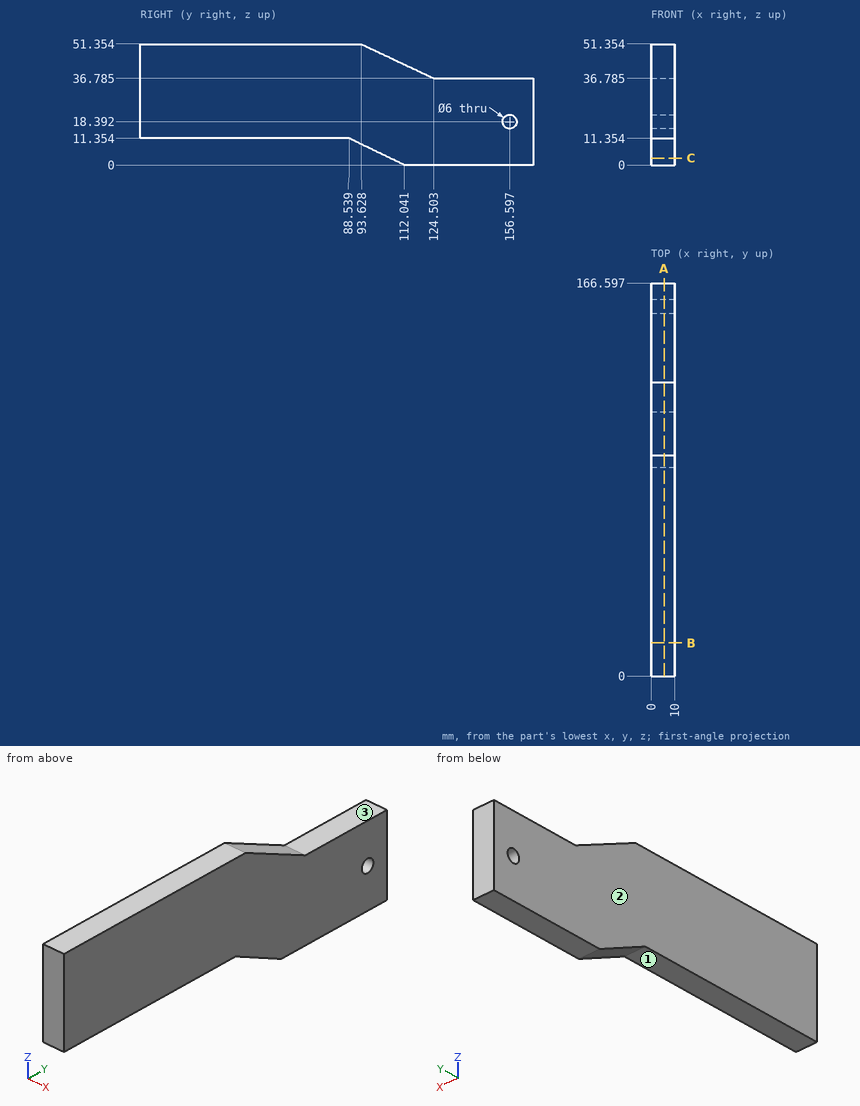
Geometry check sheet. Reference: drawing and pictorial views, mm from the part's lowest x, y, z. A direction names the side the tool comes from. Coordinates: 2 decimals unless noted, no trailing zeros. Order: outer loops, then holes, each group sorted by start corner. A loop starts at its lowest first (then second) coordinate and runs counter-clockwise, first axis right, second up. Notation, with made-up numbers: (72, 47) - (123, 47) arc R22 cw to (123, 74) - close; hole circle Ø4 at (-30.75, 71). An arc over 180 degrees is marked (long way). One line per item, written item: value.
(1) Thickness scan on probe 1 along Z at (x, y) = (4, 157) (1 decimal); probe 2 along Z at (x, y) = (5.25, 132) (1 decimal); probe 3 along Z at (x, y) = (0.75, 42.5). Record the ranges inside material, lowest first. Write a range as from..to.
Data:
probe 1: z = 0..15.4, 21.4..36.8
probe 2: z = 0..36.8
probe 3: z = 11.35..51.35
(2) Sectioned sample at B-B (y = 14). Enter the section's corners in (x, z), and give its area (3 significant figures).
Data:
outline: (0, 11.35) - (10, 11.35) - (10, 51.35) - (0, 51.35) - close
area: 400 mm^2
(3) Depth check by flat-ended pin: pin 1 Ø3 at (x, y) = (4, 51.5) entering from -Z; pin 2 Ø2 at (x, z) = (8.5, 31) entering from -Y; pin 3 Ø5 at (x, y) = (5.5, 135.5) entering from +Z (1 decimal). Enter the tip coordinate at first touch or a pass-through.
Data:
pin 1: stops at z = 11.35
pin 2: stops at y = 0
pin 3: stops at z = 36.8
(4) Sectioned sample at C-C (z = 3). Enter the section's corners in (x, y), and give its area (3 significant figures).
Data:
outline: (0, 105.83) - (10, 105.83) - (10, 166.6) - (0, 166.6) - close
area: 608 mm^2
(5) Access from +Z, -Z, +X, -X, +Y, -Y to the whole of each face (thin tool, end or side, straight path). Record for the marked faces 1, 2 and 3.
Data:
face 1: -Z, +X, -X, -Y
face 2: +Z, -Z, -X, +Y, -Y
face 3: +Z, +X, -X, +Y
(6) Sectioned sample at A-A (x = 5.5). Enter the section's corners in (y, z) (1 decimal), and give its area (3 significant figures).
Data:
outline: (0, 11.4) - (88.5, 11.4) - (112, 0) - (166.6, 0) - (166.6, 36.8) - (124.5, 36.8) - (93.6, 51.4) - (0, 51.4) - close; hole circle Ø6 at (156.6, 18.4)
area: 6,550 mm^2
